Geometry: final body of the model. Coordinates: model frame, mm. Coordinates: 2 decimals unless noted, no trailing zeros. Loops run counter-clockwise (first coordinate to the right, second up) from the corner with the lowest first, then second, coordinate; pieces in that order, holes last. Notation, with made-up numbers: M -25,-7.5 L 1,-7.5 A24 cw 1,5.5 Z; hole C 47.25,-0.75 d4. An arc over 180 degrees is marked long. Write each question's results on one line, items separated by ' | '. Start each with the question number.
from build123d import *

# Parameters (mm, degrees)
SKETCH1_W                    = 3.175
SKETCH1_H                    = 12.7
MAIN_EXTRUDE_DEPTH           = 3.175
SKETCH8_R                    = 1.5
SKETCH8_W                    = 3.175
SKETCH8_H                    = 31.877
MOUNT_HOLES_DEPTH            = 4.175
DOOR_SLOTS_DEPTH             = 4.175
SKETCH10_R                   = 1.5
DOOR_GUIDE_MOUNT_HOLES_DEPTH = 4.175
SKETCH12_R                   = 1.5
EXTENSION_CLIP_HOLES_DEPTH   = 4.175
EXTENSION_CENTER_CUT_DEPTH   = 4.175
SKETCH17_W                   = 30.1
SKETCH17_H                   = 16.51
SKETCH17_W_2                 = 25.230666667
SKETCH17_H_2                 = 5.588
NOSEPOKES_SCOPED_DEPTH       = 4.175


with BuildPart() as part:
    # Sketch1 → Main Extrude (new body)
    with BuildSketch(Plane.XY):
        Polygon((-243.84, -134.112), (-189.653333333, -134.112), (-189.653333333, -139.7), (-135.466666667, -139.7), (-135.466666667, -134.112), (-81.28, -134.112), (-81.28, -139.7), (-27.093333333, -139.7), (-27.093333333, -134.112), (27.093333333, -134.112), (27.093333333, -139.7), (81.28, -139.7), (81.28, -134.112), (135.466666667, -134.112), (135.466666667, -139.7), (189.653333333, -139.7), (189.653333333, -134.112), (243.84, -134.112), (243.84, -139.7), (298.026666667, -139.7), (298.026666667, -134.112), (352.213333333, -134.112), (352.213333333, -139.7), (406.4, -139.7), (406.4, 139.7), (381, 139.7), (381, 127), (377.825, 127), (377.825, 139.7), (-377.825, 139.7), (-377.825, 127), (-381, 127), (-381, 139.7), (-406.4, 139.7), (-406.4, -139.7), (-352.213333333, -139.7), (-352.213333333, -134.112), (-298.026666667, -134.112), (-298.026666667, -139.7), (-243.84, -139.7), align=None)
        with Locations((-379.4125, -120.65)):
            Rectangle(SKETCH1_W, SKETCH1_H, mode=Mode.SUBTRACT)
        with Locations((-379.4125, -95.25)):
            Rectangle(SKETCH1_W, SKETCH1_H, mode=Mode.SUBTRACT)
        with Locations((379.4125, 82.55)):
            Rectangle(SKETCH1_W, SKETCH1_H, mode=Mode.SUBTRACT)
        with Locations((379.4125, 57.15)):
            Rectangle(SKETCH1_W, SKETCH1_H, mode=Mode.SUBTRACT)
        with Locations((379.4125, 31.75)):
            Rectangle(SKETCH1_W, SKETCH1_H, mode=Mode.SUBTRACT)
        with Locations((379.4125, 6.35)):
            Rectangle(SKETCH1_W, SKETCH1_H, mode=Mode.SUBTRACT)
        with Locations((379.4125, -19.05)):
            Rectangle(SKETCH1_W, SKETCH1_H, mode=Mode.SUBTRACT)
        with Locations((379.4125, -44.45)):
            Rectangle(SKETCH1_W, SKETCH1_H, mode=Mode.SUBTRACT)
        with Locations((379.4125, -69.85)):
            Rectangle(SKETCH1_W, SKETCH1_H, mode=Mode.SUBTRACT)
        with Locations((379.4125, -95.25)):
            Rectangle(SKETCH1_W, SKETCH1_H, mode=Mode.SUBTRACT)
        with Locations((379.4125, -120.65)):
            Rectangle(SKETCH1_W, SKETCH1_H, mode=Mode.SUBTRACT)
        with Locations((-379.4125, -69.85)):
            Rectangle(SKETCH1_W, SKETCH1_H, mode=Mode.SUBTRACT)
        with Locations((-379.4125, -44.45)):
            Rectangle(SKETCH1_W, SKETCH1_H, mode=Mode.SUBTRACT)
        with Locations((-379.4125, -19.05)):
            Rectangle(SKETCH1_W, SKETCH1_H, mode=Mode.SUBTRACT)
        with Locations((-379.4125, 6.35)):
            Rectangle(SKETCH1_W, SKETCH1_H, mode=Mode.SUBTRACT)
        with Locations((-379.4125, 31.75)):
            Rectangle(SKETCH1_W, SKETCH1_H, mode=Mode.SUBTRACT)
        with Locations((-379.4125, 57.15)):
            Rectangle(SKETCH1_W, SKETCH1_H, mode=Mode.SUBTRACT)
        with Locations((-379.4125, 82.55)):
            Rectangle(SKETCH1_W, SKETCH1_H, mode=Mode.SUBTRACT)
        with Locations((-379.4125, 107.95)):
            Rectangle(SKETCH1_W, SKETCH1_H, mode=Mode.SUBTRACT)
        with Locations((379.4125, 107.95)):
            Rectangle(SKETCH1_W, SKETCH1_H, mode=Mode.SUBTRACT)
    extrude(amount=MAIN_EXTRUDE_DEPTH)

    # Sketch8 → Mount Holes (cut, through all)
    with BuildSketch(Plane.XY.offset(3.175)):
        with Locations((-393.7, -120.65)):
            Circle(SKETCH8_R)
        with Locations((393.7, -120.65)):
            Circle(SKETCH8_R)
        with Locations((-382.5875, 12.319)):
            Rectangle(SKETCH8_W, SKETCH8_H)
        with Locations((382.5875, 12.319)):
            Rectangle(SKETCH8_W, SKETCH8_H)
    extrude(amount=-MOUNT_HOLES_DEPTH, mode=Mode.SUBTRACT)

    # Sketch3 → Door Slots (cut, through all)
    with BuildSketch(Plane.XY.offset(3.175)):
        Polygon((-88.7095, 126.492), (-92.6465, 126.492), (-92.6465, 82.042), (-96.52, 82.042), (-96.52, 10.3505), (-106.553, 10.3505), (-106.553, 0.8255), (-96.52, 0.8255), (-96.52, -134.112), (-84.836, -134.112), (-84.836, 0.8255), (-74.803, 0.8255), (-74.803, 10.3505), (-84.836, 10.3505), (-84.836, 82.042), (-88.7095, 82.042), align=None)
        Polygon((92.6465, 126.492), (88.7095, 126.492), (88.7095, 82.042), (84.836, 82.042), (84.836, 10.3505), (74.803, 10.3505), (74.803, 0.8255), (84.836, 0.8255), (84.836, -134.112), (96.52, -134.112), (96.52, 0.8255), (106.553, 0.8255), (106.553, 10.3505), (96.52, 10.3505), (96.52, 82.042), (92.6465, 82.042), align=None)
    extrude(amount=-DOOR_SLOTS_DEPTH, mode=Mode.SUBTRACT)

    # Sketch10 → Door Guide Mount Holes (cut, through all)
    with BuildSketch(Plane.XY.offset(3.175)):
        with Locations((-101.678, 127.492)):
            Circle(SKETCH10_R)
        with Locations((-79.678, 127.492)):
            Circle(SKETCH10_R)
        with Locations((79.678, 127.492)):
            Circle(SKETCH10_R)
        with Locations((101.678, 127.492)):
            Circle(SKETCH10_R)
    extrude(amount=-DOOR_GUIDE_MOUNT_HOLES_DEPTH, mode=Mode.SUBTRACT)

    # Sketch12 → Extension Clip Holes (cut, through all)
    with BuildSketch(Plane.XY.offset(3.175)):
        with Locations((-246.507, 20.193)):
            Circle(SKETCH12_R)
        with Locations((-246.507, 4.445)):
            Circle(SKETCH12_R)
        with Locations((-221.107, 4.445)):
            Circle(SKETCH12_R)
        with Locations((-221.107, 20.193)):
            Circle(SKETCH12_R)
        with Locations((-243.332, 133.35)):
            Circle(SKETCH12_R)
        with Locations((-224.282, 133.35)):
            Circle(SKETCH12_R)
        with Locations((224.282, 133.35)):
            Circle(SKETCH12_R)
        with Locations((243.332, 133.35)):
            Circle(SKETCH12_R)
        with Locations((221.107, 20.193)):
            Circle(SKETCH12_R)
        with Locations((221.107, 4.445)):
            Circle(SKETCH12_R)
        with Locations((246.507, 4.445)):
            Circle(SKETCH12_R)
        with Locations((246.507, 20.193)):
            Circle(SKETCH12_R)
    extrude(amount=-EXTENSION_CLIP_HOLES_DEPTH, mode=Mode.SUBTRACT)

    # Sketch11_3 → Extension Center Cut (cut, through all)
    with BuildSketch(Plane.XY.offset(3.175)):
        Polygon((-232.2195, 127), (-232.2195, 139.7), (-406.4, 139.7), (-406.4, -139.7), (-235.3945, -139.7), (-235.3945, -127), (-232.2195, -127), (-232.2195, -114.3), (-235.3945, -114.3), (-235.3945, -101.6), (-232.2195, -101.6), (-232.2195, -88.9), (-235.3945, -88.9), (-235.3945, -76.2), (-232.2195, -76.2), (-232.2195, -63.5), (-235.3945, -63.5), (-235.3945, -50.8), (-232.2195, -50.8), (-232.2195, -38.1), (-235.3945, -38.1), (-235.3945, -25.4), (-232.2195, -25.4), (-232.2195, -12.7), (-235.3945, -12.7), (-235.3945, 0), (-232.2195, 0), (-232.2195, 12.7), (-235.3945, 12.7), (-235.3945, 25.4), (-232.2195, 25.4), (-232.2195, 38.1), (-235.3945, 38.1), (-235.3945, 50.8), (-232.2195, 50.8), (-232.2195, 63.5), (-235.3945, 63.5), (-235.3945, 76.2), (-232.2195, 76.2), (-232.2195, 88.9), (-235.3945, 88.9), (-235.3945, 101.6), (-232.2195, 101.6), (-232.2195, 114.3), (-235.3945, 114.3), (-235.3945, 127), align=None)
        Polygon((406.4, 139.7), (232.2195, 139.7), (232.2195, 127), (235.3945, 127), (235.3945, 114.3), (232.2195, 114.3), (232.2195, 101.6), (235.3945, 101.6), (235.3945, 88.9), (232.2195, 88.9), (232.2195, 76.2), (235.3945, 76.2), (235.3945, 63.5), (232.2195, 63.5), (232.2195, 50.8), (235.3945, 50.8), (235.3945, 38.1), (232.2195, 38.1), (232.2195, 25.4), (235.3945, 25.4), (235.3945, 12.7), (232.2195, 12.7), (232.2195, 0), (235.3945, 0), (235.3945, -12.7), (232.2195, -12.7), (232.2195, -25.4), (235.3945, -25.4), (235.3945, -38.1), (232.2195, -38.1), (232.2195, -50.8), (235.3945, -50.8), (235.3945, -63.5), (232.2195, -63.5), (232.2195, -76.2), (235.3945, -76.2), (235.3945, -88.9), (232.2195, -88.9), (232.2195, -101.6), (235.3945, -101.6), (235.3945, -114.3), (232.2195, -114.3), (232.2195, -127), (235.3945, -127), (235.3945, -139.7), (406.4, -139.7), align=None)
    extrude(amount=-EXTENSION_CENTER_CUT_DEPTH, mode=Mode.SUBTRACT)

    # Sketch17 → nosepokes_scoped (cut, through all)
    with BuildSketch(Plane.XY.offset(3.175)):
        with Locations((42.291, -110.109)):
            Rectangle(SKETCH17_W, SKETCH17_H)
        with Locations((-42.164, -110.109)):
            Rectangle(SKETCH17_W, SKETCH17_H)
        with Locations((-39.708666667, -136.906)):
            Rectangle(SKETCH17_W_2, SKETCH17_H_2)
    extrude(amount=-NOSEPOKES_SCOPED_DEPTH, mode=Mode.SUBTRACT)


solid = part.part
Item 1: Ray query, L1, parallel to X at y = 62, z = 2.95; L2, parallel to X at y = -61.5, z = 2.3; L3, parallel to X at y = -110, z = 0.25. Return the intervals inside material, ascending. Write a range as [from, to].
Item 2: Section B-B, the plane x = -39.5. Return loops of the section in (y, z) (3 decimals), plus the area to 3 significant figures.
Item 3: Section D-D, the plane z = 1.8. Count the separate pieces of the cut face and the enclosed holes in it, plus the area to 3 significant figures.
Item 4: Pull-direction query (Z, two-part tool) for faces 1 (the flat face through (-3, 2, 3.175)), 2 (the flat face through (-3, 2, 0)); classes: released by +Z, released by -Z, zero draft, split by the parting line, or undercut.
Item 5: Section C-C, the plane x = 114. Return loops of the section in (y, z) (3 decimals).
Item 6: Contact query for flat-ended pins moving along their axis: P1, Ø1.6, axis at y = 6.5, z = 1.5, coming from the +X side; P2, Ø1.6, axis at y = -137.5, z = 1.5, coming from the -X side; P3, Ø1, axis at y = -137.5, z = 1.5, coming from the +X side. Output: stop coordinate, or through.
Item 7: Section A-A, the plane y = -107. Return loops of the section in (x, z) (1 decimal), plus the area to 3 significant figures.
Solutions:
1) L1: x = [-232.22, -96.52], [-84.84, 84.84], [96.52, 232.22] | L2: x = [-235.39, -96.52], [-84.84, 84.84], [96.52, 235.39] | L3: x = [-235.39, -96.52], [-84.84, -57.21], [-27.11, 27.24], [57.34, 84.84], [96.52, 235.39]
2) outline: M -134.112,0 L -118.364,0 L -118.364,3.175 L -134.112,3.175 Z; M -101.854,0 L 139.7,0 L 139.7,3.175 L -101.854,3.175 Z | area: 817 mm²
3) separate pieces: 1 | enclosed holes: 12 | area: 122,000 mm²
4) face 1: released by +Z | face 2: released by -Z
5) outline: M -134.112,0 L 139.7,0 L 139.7,3.175 L -134.112,3.175 Z
6) P1: stops at x = 232.22 | P2: stops at x = -189.65 | P3: stops at x = 189.65
7) outline: M -235.4,0 L -96.5,0 L -96.5,3.2 L -235.4,3.2 Z; M -84.8,0 L -57.2,0 L -57.2,3.2 L -84.8,3.2 Z; M -27.1,0 L 27.2,0 L 27.2,3.2 L -27.1,3.2 Z; M 57.3,0 L 84.8,0 L 84.8,3.2 L 57.3,3.2 Z; M 96.5,0 L 235.4,0 L 235.4,3.2 L 96.5,3.2 Z | area: 1,230 mm²
